For this review, use the dimensioned drawing (mm, ordinates from the lowest corner) and the shaded views. A direction names the side the tool comes from. Round coordinates to 2 decimals unless told otherwise and drop trailing zeros. Loops run counter-clockwise (first coordinate to the right, second up) from the corner with the lowest first, then second, coordinate; pieces in that order, holes last. Notation, with made-up numbers: (18.5, 12.5) -> (74.5, 12.5) arc R5 ccw to (74.5, 18.5) -> close; hole circle Ø5 at (-6.75, -18.75). An arc over 180 degrees is marked (long way). Write each question's results on one line, items separated by ' | '.
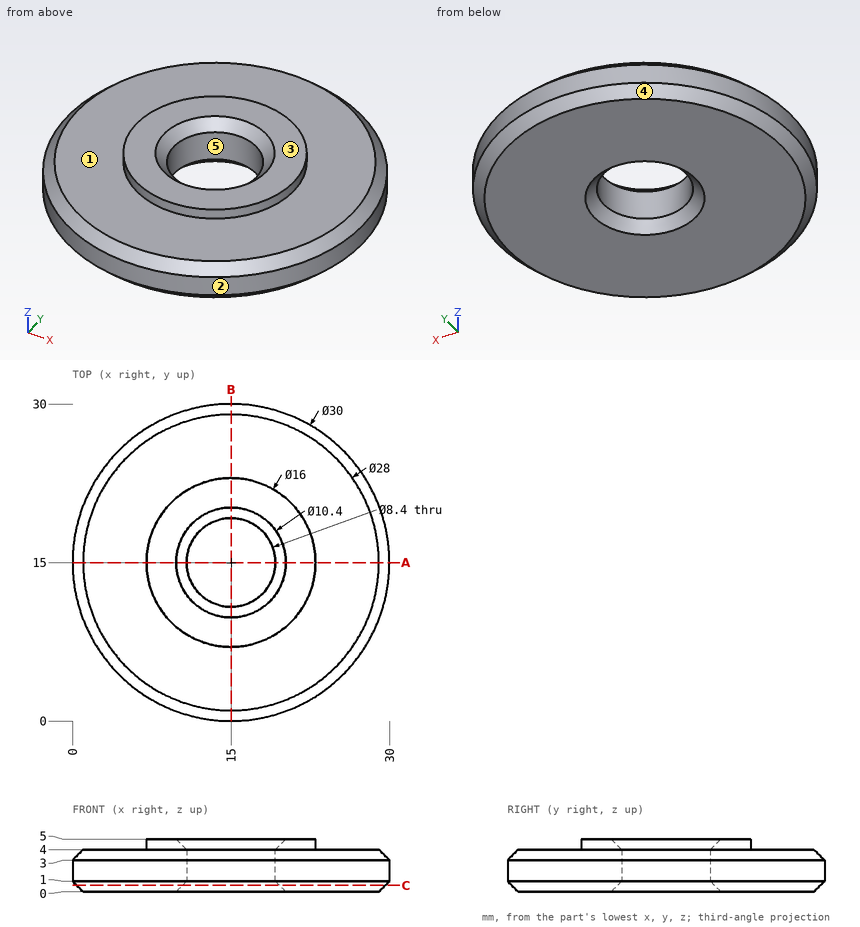
1. Tool access review of the marked faces 1 and 2: name each direction out of +Z, -Z, +X, -X, +Y, -Y from which nothing blocks a thin tool from reaching the whole face with its end or side.
Values found:
face 1: +Z | face 2: +Z, -Z
2. Draft analysis for pull direction Y (two halves, no side actions). For the marked faces 3, 4 and 5, state which applies: released by +Y, released by -Y, zero draft, split by the parting line, or undercut.
Values found:
face 3: zero draft | face 4: split by the parting line | face 5: undercut
3. To check wall thickness, follow probe 1 along Y at (x, z) = (15, 2.15); probe 2 along Z at (x, y) = (12.75, 5.75); probe 3 along Y at (x, z) = (17.75, 3.2). State the ranges of each line that lie inside material, in increasing order.
Values found:
probe 1: y = 0 to 10.8, 19.2 to 30 | probe 2: z = 0 to 4 | probe 3: y = 0.46 to 11.83, 18.17 to 29.54
4. Consider section C-C (z = 0.6). State the section outline as (x, y) points, plus the area to 3 significant figures.
Values found:
outline: circle Ø29.2 at (15, 15); hole circle Ø9.2 at (15, 15) | area: 603 mm2
5. For pin 1 (1.5 mm diameter, centred on y = 18, z = 4.5, fed in from +X); pin 2 (3 mm diameter, centred on x = 6.5, z = 4, fed in from +Y); pin 3 (1 mm diameter, centred on y = 12, z = 1, fed in from -X), all flat-tipped, find the tip position at first contact; note any pin that passes through.
Values found:
pin 1: stops at x = 28.95 | pin 2: stops at y = 28.06 | pin 3: stops at x = 0.21
6. Consider section A-A (y = 15). State the section outline as (x, z) points, plus the area to 3 significant figures.
Values found:
outline: (0, 1) -> (1, 0) -> (9.8, 0) -> (10.8, 1) -> (10.8, 4) -> (9.8, 5) -> (7, 5) -> (7, 4) -> (1, 4) -> (0, 3) -> close; (19.2, 1) -> (20.2, 0) -> (29, 0) -> (30, 1) -> (30, 3) -> (29, 4) -> (23, 4) -> (23, 5) -> (20.2, 5) -> (19.2, 4) -> close | area: 90.0 mm2
